```python
from build123d import *

# Parameters (mm, degrees)
BOSS_EXTRUDE1_DEPTH = 6.35
SKETCH2_W           = 139.7
SKETCH2_H           = 25.4
CUT_EXTRUDE1_DEPTH  = 503.934431611
SKETCH4_R           = 1.5875
SKETCH4_R_2         = 1.5
SKETCH4_R_3         = 25.4
CUT_EXTRUDE2_DEPTH  = 503.934431611


with BuildPart() as part:
    # Sketch1 → Boss-Extrude1 (new body)
    with BuildSketch(Plane.XY):
        with BuildLine():
            Line((25.4, 0), (330.2, 0))
            ThreePointArc((330.2, 0), (348.160512242, 7.439487758), (355.6, 25.4))
            Line((355.6, 25.4), (355.6, 330.2))
            ThreePointArc((355.6, 330.2), (348.160512242, 348.160512242), (330.2, 355.6))
            Line((330.2, 355.6), (25.4, 355.6))
            ThreePointArc((25.4, 355.6), (7.439487758, 348.160512242), (0, 330.2))
            Line((0, 330.2), (0, 25.4))
            ThreePointArc((0, 25.4), (7.439487758, 7.439487758), (25.4, 0))
        make_face()
    extrude(amount=BOSS_EXTRUDE1_DEPTH)

    # Sketch2 → Cut-Extrude1 (cut, through all)
    with BuildSketch(Plane(origin=(0, 0, 0), x_dir=(-1, 0, 0), z_dir=(0, 0, -1))):
        with Locations((-120.65, 342.9)):
            Rectangle(SKETCH2_W, SKETCH2_H)
        with Locations((-120.65, 12.7)):
            Rectangle(SKETCH2_W, SKETCH2_H)
    extrude(amount=-CUT_EXTRUDE1_DEPTH, mode=Mode.SUBTRACT)

    # Sketch4 → Cut-Extrude2 (cut, through all)
    with BuildSketch(Plane(origin=(0, 0, 0), x_dir=(-1, 0, 0), z_dir=(0, 0, -1))):
        with Locations((-279.42318149, 84.573787042)):
            Circle(SKETCH4_R)
        with Locations((-278.15318149, 132.833787042)):
            Circle(SKETCH4_R)
        with Locations((-196.87318149, 84.573787042)):
            Circle(SKETCH4_R)
        with Locations((-203.22318149, 132.833787042)):
            Circle(SKETCH4_R)
        with Locations((-288.258815439, 176.472066732)):
            Circle(SKETCH4_R_2)
        with Locations((-220.058815439, 176.472066732)):
            Circle(SKETCH4_R_2)
        with Locations((-194.758815439, 176.472066732)):
            Circle(SKETCH4_R_2)
        with Locations((-288.258815439, 282.772066732)):
            Circle(SKETCH4_R_2)
        with Locations((-194.758815439, 282.772066732)):
            Circle(SKETCH4_R_2)
        with Locations((-127, 215.9)):
            Circle(SKETCH4_R_3)
        with Locations((-127, 139.7)):
            Circle(SKETCH4_R_3)
    extrude(amount=-CUT_EXTRUDE2_DEPTH, mode=Mode.SUBTRACT)


solid = part.part
```
Check sheet for the modelled part. Datum: model origin and axes. Units: mm. Round coordinates to 2 decimals unless told otherwise and drop trailing zeros. Loops run counter-clockwise (first coordinate to the right, second up) from the corner with the lowest first, then second, coordinate; pieces in that order, holes last. Notation, with made-up numbers: (-10, 4) - (47, 4) arc R7 ccw to (47, 15) - close; hole circle Ø5 at (-18, 15). An arc over 180 degrees is marked (long way). Answer as a JSON object with one key per item and string values. Group by question number.
Q1. Gauge pin test, flat ends, axial feed: P1, Ø5, axis at x = 278.15, y = 132.83, coming from the -Z side; P2, Ø1.9, axis at y = 11, z = 4.5, coming from the +X side; P3, Ø3, axis at x = 128, z = 4.5, coming from the -Y side; P4, Ø1.8, axis at x = 288.26, y = 282.77, coming from the -Z side. Record the tip position at first contact, or that the pin passes through.
Q2. Mould release check, pull along Y, two halves, no side actions. Record for faces 1 (the face through (113.35, 161.12, 3.13)), 2 (the face through (347.96, 7.24, 3.13)), 3 (the face through (348.36, 347.96, 3.13)): released by +Y, released by -Y, zero draft, split by the parting line, or undercut.
Q3. Scan lines: line 1 along X through (y, z) = (24, 3.5); line 2 along X through (y, z) = (176.5, 2); line 3 along Y through (x, z) = (287.5, 5). Record each from-to range of solid material in increasing order. Write a range as [from, to].
Q4. Sectioned sample at B-B, the plane y = 139.7. Enter the section's corners in (x, z), plus the area to 3 significant figures.
Q5. Sectioned sample at C-C, the plane z = 4.25. Count the separate pieces of the cut face and the enclosed holes in it, plus the area to 3 significant figures.
Q6. Sectioned sample at A-A, the plane x = 127. Enter the section's corners in (y, z).
Solution:
{
 "1": {"P1": "stops at z = 0", "P2": "stops at x = 351.75", "P3": "stops at y = 25.4", "P4": "passes through"},
 "2": {"face 1": "undercut", "face 2": "released by -Y", "face 3": "released by +Y"},
 "3": {"line 1": "x = [0.04, 50.8], [190.5, 355.56]", "line 2": "x = [0, 193.26], [196.26, 218.56], [221.56, 286.76], [289.76, 355.6]", "line 3": "y = [0, 175.18], [177.77, 281.48], [284.07, 355.6]"},
 "4": {"outline": "(0, 0) - (101.6, 0) - (101.6, 6.35) - (0, 6.35) - close; (152.4, 0) - (355.6, 0) - (355.6, 6.35) - (152.4, 6.35) - close", "area": "1,940 mm²"},
 "5": {"separate pieces": "1", "enclosed holes": "11", "area": "115,000 mm²"},
 "6": {"outline": "(25.4, 0) - (114.3, 0) - (114.3, 6.35) - (25.4, 6.35) - close; (165.1, 0) - (190.5, 0) - (190.5, 6.35) - (165.1, 6.35) - close; (241.3, 0) - (330.2, 0) - (330.2, 6.35) - (241.3, 6.35) - close"}
}
